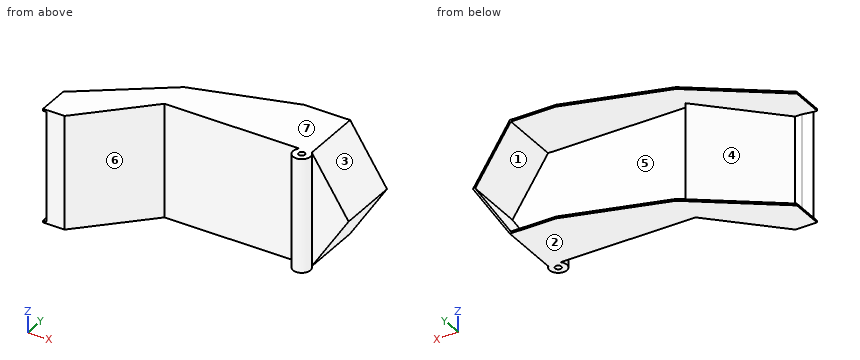
from build123d import *

# Parameters (mm, degrees)
BOSS_EXTRUDE1_DEPTH = 100
SHELL1_T            = -3
SKETCH2_W           = 3
SKETCH2_H           = 179
CUT_EXTRUDE1_DEPTH  = 97
CUT_EXTRUDE2_DEPTH  = 367.367302034
SKETCH4_R           = 5
BOSS_EXTRUDE2_DEPTH = 185
BOSS_EXTRUDE3_REACH = 368.367
SHELL2_START        = -182
SHELL2_DEPTH        = 179
SKETCH6_W           = 8.912859495
SKETCH6_H           = 179
CUT_EXTRUDE3_DEPTH  = 10
CHAMFER1_SIZE       = 4
CHAMFER1_SIZE_2     = 22.685127278
BOSS_EXTRUDE4_REACH = 366.862


# Read off the part's stored shape, not the designer's step: Shell2
with BuildPart() as part:
    # Sketch1 → Boss-Extrude1 (new body)
    with BuildSketch(Plane(origin=(0, 0, 0), x_dir=(1, 0, 0), z_dir=(0, 1, 0))):
        Polygon((240, 185), (300, 92.5), (240, 0), (0, 0), (0, 185), align=None)
    extrude(amount=BOSS_EXTRUDE1_DEPTH)

    # Shell1
    shell1_openings = [part.faces().sort_by_distance(p)[0] for p in [
        (135.555555556, 100, -92.5),
    ]]
    offset(amount=SHELL1_T, openings=shell1_openings, kind=Kind.INTERSECTION)

    # Sketch2 → Cut-Extrude1 (cut)
    with BuildSketch(Plane(origin=(0, 100, 0), x_dir=(1, 0, 0), z_dir=(0, 1, 0))):
        with Locations((1.5, 92.5)):
            Rectangle(SKETCH2_W, SKETCH2_H)
    extrude(amount=-CUT_EXTRUDE1_DEPTH, mode=Mode.SUBTRACT)

    # Sketch3 → Cut-Extrude2 (cut, through all)
    with BuildSketch(Plane.XY):
        Polygon((0, 100), (0, 51.158972719), (164.988073302, 100), align=None)
    extrude(amount=-CUT_EXTRUDE2_DEPTH, mode=Mode.SUBTRACT)

    # Sketch4 → Boss-Extrude2 (add)
    with BuildSketch(Plane.XY):
        with BuildLine():
            Line((220, 0), (240, 0))
            ThreePointArc((240, 0), (230, -24.142135624), (220, 0))
        make_face()
        with Locations((230, -10)):
            Circle(SKETCH4_R, mode=Mode.SUBTRACT)
    extrude(amount=-BOSS_EXTRUDE2_DEPTH)

    # Boss-Extrude3: up to this face of the body (flat: up to its plane)
    boss_extrude3_end = Plane(part.part.faces().sort_by_distance((135.447130894, 41.883724311, -185))[0])
    # Sketch5 → Boss-Extrude3 (add, up to the picked face)
    with BuildSketch(Plane.XY, mode=Mode.PRIVATE) as boss_extrude3_sk1:
        Polygon((0, 51.158972719), (-135, -47.5), (-135, -100), (-100, -100), (0, 0), align=None)
    boss_extrude3_tool1 = split(extrude(boss_extrude3_sk1.sketch, amount=-BOSS_EXTRUDE3_REACH, mode=Mode.PRIVATE), bisect_by=boss_extrude3_end, keep=Keep.BOTH, mode=Mode.PRIVATE)
    add(boss_extrude3_tool1.solids().sort_by(Axis((-69.900259, -32.775799, 0), (0, 0, -1)))[0])

    # Shell2 outline → Shell2 (cut)
    with BuildSketch(Plane.XY.offset(SHELL2_START)):
        Polygon((0, 48.030284306), (-7.196033451, 45.900059624), (-135, -47.5), (-135, -97), (-101.242640687, -97), (-1.242640687, 3), (0, 3), align=None)
    extrude(amount=SHELL2_DEPTH, mode=Mode.SUBTRACT)

    # Sketch6 → Cut-Extrude3 (cut)
    with BuildSketch(Plane(origin=(-24.371197118, 33.348326263, 0), x_dir=(0.8073765164894111, 0.5900365756641057, 0), z_dir=(-0.5900365756641056, 0.8073765164894111, 0))):
        with Locations((25.729235331, 92.5)):
            Rectangle(SKETCH6_W, SKETCH6_H)
    extrude(amount=-CUT_EXTRUDE3_DEPTH, mode=Mode.SUBTRACT)

    # Chamfer1
    # the kernel refuses this chamfer: 22.685127278, 4 mm, written as the material it takes off along each edge
    with BuildSketch(Plane(origin=(-135, -97, -182), x_dir=(-0.21013876076735197, -0.9776715712462758, 0), z_dir=(0, 0, 1))) as chamfer1_piece_1:
        Polygon((CHAMFER1_SIZE * 0.977671571246, CHAMFER1_SIZE * 0.210138760767), (-CHAMFER1_SIZE_2 * 0.210138760772, CHAMFER1_SIZE_2 * 0.977671571267), (0, 0), align=None)
    extrude(amount=179, mode=Mode.SUBTRACT)

    # Sketch8 → Boss-Extrude4 (add, up to next)
    with BuildSketch(Plane.XY.offset(-182), mode=Mode.PRIVATE) as boss_extrude4_sk1:
        Polygon((-1.242640687, 3), (8.757359313, 13), (8.757359313, 3), align=None)
    boss_extrude4_tool1 = extrude(boss_extrude4_sk1.sketch, amount=BOSS_EXTRUDE4_REACH, mode=Mode.PRIVATE) - part.part
    add(boss_extrude4_tool1.solids().sort_by_distance((5.424026, 6.333333, -182))[0])


solid = part.part
Part model, mm, in its own coordinate system. Face numbers are marked on the shaded views. A direction names the side the tool comes from. Coordinates: 2 decimals unless noted, no trailing zeros. Loops run counter-clockwise (first coordinate to the right, second up) from the corner with the lowest first, then second, coordinate; pieces in that order, holes last. Notation, with made-up numbers: (85, 11) -> (134, 11) arc R12 ccw to (134, 27) -> close; hole circle Ø8 at (-20, 40). An arc over 180 degrees is marked (long way). Use a Markdown table: item, result. Add a question column.
Item 1: Band-saw the part on D-D on z = -19. Write the cut outline in (x, y).
Item 2: Which spindle directions (+Z, -Z, +X, -X, +Y, -Y) get a long thin tool onto all of the face, cutting with end or side? Do the marked faces 4, 5, 6 and 7. Say none if no direction does.
Item 3: Flat gauge pins, fed straight in: P1, Ø3, axis at y = -8.5, z = -148, coming from the +X side; P2, Ø8, axis at x = 252.5, z = -113.5, coming from the +Y side; P3, Ø9, axis at x = 230, y = -10, coming from the +Z side; P4, Ø5.5, axis at x = -106, z = -89.5, coming from the +Y side. Where does each tip first touch, or does it go through?
Item 4: Band-saw the part on C-C on y = -10. Write the cut outline in (x, z), plus the area to 3 significant figures.
Item 5: Probe probe 1 along Z at (x, y) = (154.5, 11.5); probe 2 along Y at (x, z) = (230, -142); probe 3 along Y at (x, z) = (71, -100.5). List the from-to ranges inside material, lowest first.
Item 6: Band-saw the part on B-B on x = 176. Write the cut outline in (y, z), plus the area to 3 significant figures.
Item 7: Band-saw the part on A-A on x = 230. Write the cut outline in (y, z).
Item 8: Pull direction Z, two halves, no side cores. Call the marked faces 1, 2 and 3: +Z half, -Z half, draft (parallel to the pull), parting line (faces both ways), or undercut.
Geometry says:
| question | item | result |
|---|---|---|
| 1 | outline | (-129.33, -100) -> (-100, -100) -> (0, 0) -> (220, 0) arc R14.14 ccw (long way) to (240, 0) -> (252.32, 0) -> (252.32, 100) -> (248.75, 100) -> (248.75, 3) -> (8.76, 3) -> (8.76, 13) -> (-101.24, -97) -> (-112.31, -97) -> close; hole circle Ø10 at (230, -10) |
| 2 | face 4 | -X, +Y |
| 2 | face 5 | +Y |
| 2 | face 6 | +Z, -Z, -Y |
| 2 | face 7 | +Z, +X, -X, +Y, -Y |
| 3 | P1 | x = 244.14 |
| 3 | P2 | y = 3 |
| 3 | P3 | through |
| 3 | P4 | y = -97 |
| 4 | outline | (-83.69, -185) -> (-10, -185) -> (-10, 0) -> (-83.69, 0) -> (-83.69, -3) -> (-14.24, -3) -> (-14.24, -182) -> (-83.69, -182) -> close; (215.86, -185) -> (225, -185) -> (225, 0) -> (215.86, 0) -> close; (235, -185) -> (244.14, -185) -> (244.14, 0) -> (235, 0) -> close |
| 4 | area | 4,580 mm² |
| 5 | probe 1 | -185 to -182, -3 to 0 |
| 5 | probe 2 | -24.14 to -15, -5 to 3 |
| 5 | probe 3 | 0 to 3 |
| 6 | outline | (0, -185) -> (100, -185) -> (100, -182) -> (3, -182) -> (3, -3) -> (100, -3) -> (100, 0) -> (0, 0) -> close |
| 6 | area | 1,140 mm² |
| 7 | outline | (-24.14, -185) -> (-15, -185) -> (-15, 0) -> (-24.14, 0) -> close; (-5, -185) -> (100, -185) -> (100, -182) -> (3, -182) -> (3, -3) -> (100, -3) -> (100, 0) -> (-5, 0) -> close |
| 8 | face 1 | undercut |
| 8 | face 2 | -Z half |
| 8 | face 3 | +Z half |
